Drawing for the job (mm, zero at the part's lowest x, y, z). A direction names the side the tool comes from. Coordinates: 2 decimals unless noted, no trailing zeros. Loops run counter-clockwise (first coordinate to the right, second up) from the corner with the lowest first, then second, coordinate; pieces in that order, holes last. Notation, with made-up numbers: (88.25, -38.75) - (141.25, -38.75) arc R23 ccw to (141.25, -9.75) - close; hole circle Ø11 at (24, -10.75). An arc over 180 degrees is marked (long way). One line per item, written item: value.
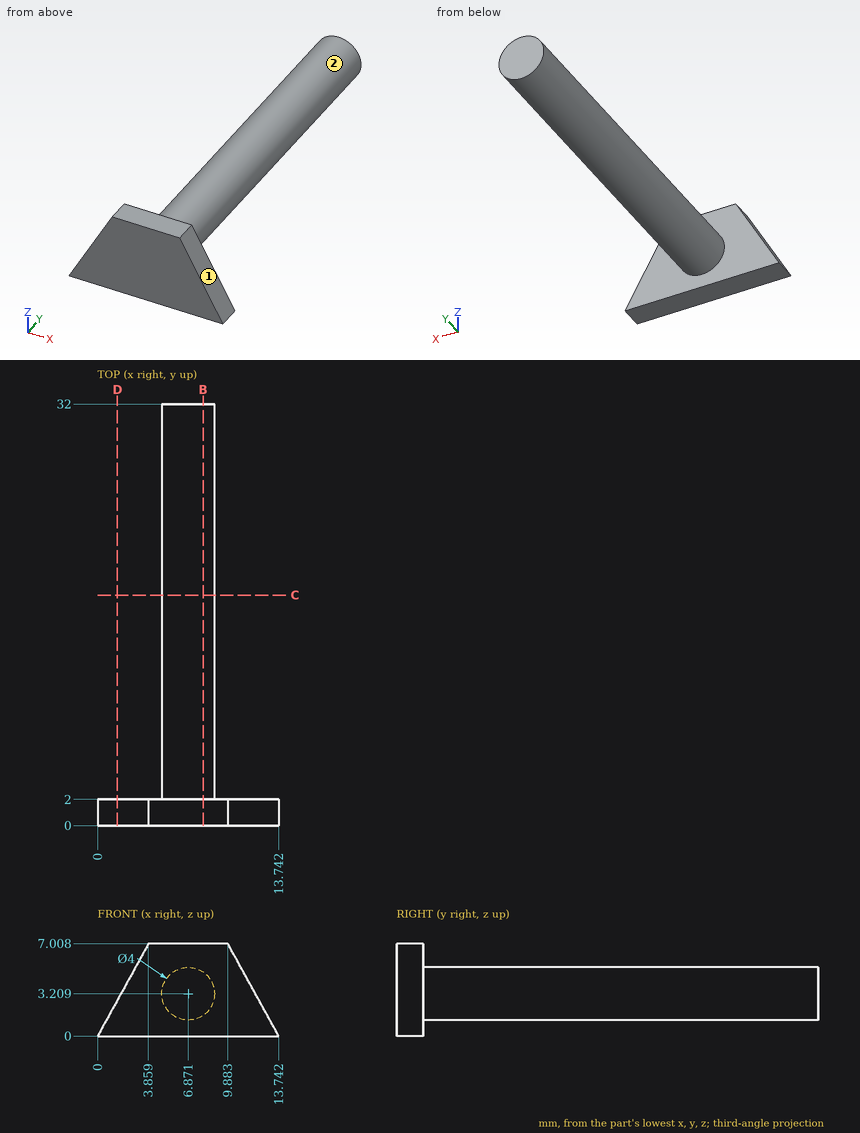
Item 1: Tool access for the marked faces 1 and 2: list every direction of +Z, -Z, +X, -X, +Y, -Y with a clear straight run to the whole face (end or side of a thin tool).
Check result:
face 1: +Z, +X, +Y, -Y
face 2: +Y
Item 2: Cut at D-D, the plane x = 1.5. Write the cut outline in (y, z).
Check result:
outline: (0, 0) - (2, 0) - (2, 2.72) - (0, 2.72) - close
Item 3: Cut at B-B, the plane x = 8. Write the cut outline in (y, z), then the cut area to 3 significant figures.
Check result:
outline: (0, 0) - (2, 0) - (2, 1.56) - (32, 1.56) - (32, 4.86) - (2, 4.86) - (2, 7.01) - (0, 7.01) - close
area: 113 mm^2
Item 4: Cut at C-C, the plane y = 17.5. Write the cut outline in (x, z), then the cut area to 3 significant figures.
Check result:
outline: circle Ø4 at (6.87, 3.21)
area: 12.6 mm^2
Item 5: Probe probe 1 along Y at (x, z) = (11, 4.5); probe 2 along X at (y, z) = (21.5, 3.5); probe 3 along X at (y, z) = (11.5, 2.5). List the from-to ranges inside material, lowest first. Write a range as from..to.
Check result:
probe 1: y = 0..2
probe 2: x = 4.89..8.85
probe 3: x = 5..8.74
Item 6: Drop flat-ended pins along their axis: P1, Ø1, axis at y = 12, z = 3.5, coming from the +X side; P2, Ø3, axis at x = 7, y = 4.5, coming from the +Z side. Give the stop position or say it passes through.
Check result:
P1: stops at x = 8.87
P2: stops at z = 5.21
